```python
from build123d import *

# Parameters (mm, degrees)
SKETCH_1_R      = 40.9
SKETCH_1_R_2    = 1.525
EXTRUDE_1_DEPTH = 5
SKETCH_3_W      = 30
SKETCH_3_H      = 5
EXTRUDE_2_DEPTH = 5


with BuildPart() as part:
    # 草图1 → 凸台-拉伸1 (new body)
    with BuildSketch(Plane(origin=(0, 0, 0), x_dir=(1, 0, 0), z_dir=(0, 1, 0))):
        with BuildLine():
            Line((-46.9, 0), (-46.9, 46.9))
            Line((-46.9, 46.9), (-16.9, 46.9))
            Line((-16.9, 46.9), (-16.9, 46.574671228))
            ThreePointArc((-16.9, 46.574671228), (-16.079234093, 44.95930534), (-14.290593047, 44.669776699))
            ThreePointArc((-14.290593047, 44.669776699), (37.88033008, -27.65303949), (-46.9, 0))
        make_face()
        Circle(SKETCH_1_R, mode=Mode.SUBTRACT)
        with Locations((-19.9, 39.130550724)):
            Circle(SKETCH_1_R_2, mode=Mode.SUBTRACT)
        with Locations((0, 43.9)):
            Circle(SKETCH_1_R_2, mode=Mode.SUBTRACT)
        with Locations((43.9, 0)):
            Circle(SKETCH_1_R_2, mode=Mode.SUBTRACT)
        with Locations((0, -43.9)):
            Circle(SKETCH_1_R_2, mode=Mode.SUBTRACT)
        with Locations((-43.9, 0)):
            Circle(SKETCH_1_R_2, mode=Mode.SUBTRACT)
        with Locations((-43.9, 39.130550724)):
            Circle(SKETCH_1_R_2, mode=Mode.SUBTRACT)
    extrude(amount=EXTRUDE_1_DEPTH)

    # 草图3 → 凸台-拉伸2 (add)
    with BuildSketch(Plane(origin=(0, 0, 0), x_dir=(1, 0, 0), z_dir=(0, 1, 0))):
        with Locations((-31.9, 49.4)):
            Rectangle(SKETCH_3_W, SKETCH_3_H)
    extrude(amount=EXTRUDE_2_DEPTH)


solid = part.part
```
Geometry: final body of the model. Coordinates: model frame, mm. Round coordinates to 2 decimals unless told otherwise and drop trailing zeros. Order: outer loops, then holes, each group sorted by start corner. A loop starts at its lowest first (then second) coordinate and runs counter-clockwise, first axis right, second up. Notation, with made-up numbers: (10.5, 36) - (26.5, 36) arc R20 ccw to (26.5, 67) - close; hole circle Ø10 at (71, -28.75). An arc over 180 degrees is marked (long way). Use CSV: the item, a comma, the result in double quotes. Start each with the question number.
Q1. Section query A-A (x = 27.5). Return loops of the section in (y, z), and give its area (3 significant figures).
Q2. First-contact query: pin 1 (1 mm diameter, centred on x = -5.5, y = 2.5, fed in from -Z). Flat tip, straight axial feed; report the tip coordinate or a pass-through.
Q3. Mould query, pull axis X, two halves, no side actions, for faces 1 (the face through (-21, 0, -36)), 2 (the face through (-0.33, 2.46, -42.41)), 3 (the face through (-46.9, 2, -26)). Classes: +X half, -X half, draft (parallel to the pull), parting line (faces both ways), or undercut.
Q4. Section query D-D (y = 1.25). Return loops of the section in (x, z) (3 decimals), and give its area (3 significant figures).
Q5. Section query C-C (x = -19.9). Return loops of the section in (y, z), and give its area (3 significant figures).
Q6. Section query B-B (z = 28). Return loops of the section in (x, y), and give its area (3 significant figures).
Q7. Material intervals for line 1 along X through (y, z) = (2.2, 0) (3 decimals); line 2 along Z through (x, y) = (-19, 3.9); line 3 along X through (y, z) = (1.35, -22.5), sorted ascending. Write a range as from..to.
Result set:
1,outline,"(0, -37.99) - (5, -37.99) - (5, -30.27) - (0, -30.27) - close; (0, 30.27) - (5, 30.27) - (5, 37.99) - (0, 37.99) - close"
1,area,"77.2 mm2"
2,pin 1,"stops at z = -46.63"
3,face 1,"draft"
3,face 2,"undercut"
3,face 3,"-X half"
4,outline,"(-46.9, -51.9) - (-16.9, -51.9) - (-16.9, -46.575) arc R2 cw to (-14.291, -44.67) arc R46.9 ccw (long way) to (-46.9, 0) - close; hole circle Ø3.05 at (-43.9, -39.131); hole circle Ø3.05 at (-43.9, 0); hole circle Ø81.8 at (0, 0); hole circle Ø3.05 at (-19.9, -39.131); hole circle Ø3.05 at (0, -43.9); hole circle Ø3.05 at (0, 43.9); hole circle Ø3.05 at (43.9, 0)"
4,area,"2,220 mm2"
5,outline,"(0, -51.9) - (5, -51.9) - (5, -40.66) - (0, -40.66) - close; (0, -37.61) - (5, -37.61) - (5, -35.73) - (0, -35.73) - close; (0, 35.73) - (5, 35.73) - (5, 42.47) - (0, 42.47) - close"
5,area,"99.3 mm2"
6,outline,"(-37.62, 0) - (-29.81, 0) - (-29.81, 5) - (-37.62, 5) - close; (29.81, 0) - (37.62, 0) - (37.62, 5) - (29.81, 5) - close"
6,area,"78.1 mm2"
7,line 1,"x = -46.9..-45.425, -42.375..-40.9, 40.9..42.375, 45.425..46.9"
7,line 2,"z = -51.9..-40.36, -37.9..-36.22, 36.22..42.88"
7,line 3,"x = -46.9..-34.15, 34.15..41.15"
